Autodesk Inventor part; units mm, degrees
ref_plane "YZ Plane" through (0, 0, 0) normal (1, 0, 0) x (0, 1, 0)
ref_plane "XZ Plane" through (0, 0, 0) normal (0, 1, 0) x (-1, 0, 0)
ref_plane "XY Plane" through (0, 0, 0) normal (0, 0, 1) x (1, 0, 0)
sketch "草圖1" plane through (0, 0, 0) normal (0, 0, 1) x (1, 0, 0)
  line L0 (0, -16.62) -> (0, 16.62) construction
  line L1 (2, -16.62) -> (2, 16.62)
  line L2 (-2, 16.62) -> (-2, -16.62)
  arc A0 (-2, -16.62) -> (2, -16.62) centre (0, -16.62) ccw
  arc A1 (2, 16.62) -> (-2, 16.62) centre (0, 16.62) ccw
  point P0 (0, 0)
  dimension "d0" = 33.24
  dimension "d1" = 4
extrude "擠出1" add sketch "草圖1" along normal blind 1
sketch "草圖2" plane through (0, 0, 1) normal (0, 0, 1) x (1, 0, 0)
  arc A0 (2, 16.62) -> (-2, 16.62) centre (0, 16.62) ccw
  circle A1 centre (0, 16.62) radius 0.75
  arc A2 (-2, -16.62) -> (2, -16.62) centre (0, -16.62) ccw
  circle A3 centre (0, -16.62) radius 0.75
  point P0 (0, 0)
  dimension "d4" = 1.5
  dimension "d5" = 1.5
extrude "擠出2" add sketch "草圖2" along normal blind 1
hole "孔1" at (0, -16.62, 1) at (0, 16.62, 1) direction (0, 0, -1) diameter 2 end through all
hole "孔2" at (0, -16.62, 1) at (0, 16.62, 1) direction (0, 0, 1) diameter 2 end through all
properties part number "連桿4"
Design review of the part built by this model. Coordinates are the model's own, in mm. Round coordinates to 2 decimals unless told otherwise and drop trailing zeros. Order: outer loops, then holes, each group sorted by start corner. A loop starts at its lowest first (then second) coordinate and runs counter-clockwise, first axis right, second up. Notation, with made-up numbers: (52.25, 69.5) - (80.25, 69.5) arc R17 ccw to (80.25, 94.5) - close; hole circle Ø9 at (61.25, -22.5). An arc over 180 degrees is marked (long way). Return JSON: item names as keys, results as strings.
Q1. Wall thickness on L1, parallel to Y at x = 0, z = 0.2; L2, parallel to Y at x = 0.25, z = 0.4; L3, parallel to X at y = 16.62, z = 0.5: over which ranges is each line inside the solid? List them lowest first. Write a range as [from, to].
Computed values:
{"L1": "y = [-18.62, -17.62], [-15.62, 15.62], [17.62, 18.62]", "L2": "y = [-18.6, -17.59], [-15.65, 15.65], [17.59, 18.6]", "L3": "x = [-2, -1], [1, 2]"}
Q2. Consider section A-A on x = 0. Write out the cut boundary in (y, z).
Computed values:
{"outline": "(-18.62, 0) - (-17.62, 0) - (-17.62, 1) - (-18.62, 1) - close; (-15.62, 0) - (15.62, 0) - (15.62, 1) - (-15.62, 1) - close; (17.62, 0) - (18.62, 0) - (18.62, 1) - (17.62, 1) - close"}
Q3. Consider section B-B on z = 0.2. Write out the cut boundary in (x, y), plus the area to 3 significant figures.
Computed values:
{"outline": "(-2, -16.62) arc R2 ccw to (2, -16.62) - (2, 16.62) arc R2 ccw to (-2, 16.62) - close; hole circle Ø2 at (0, -16.62); hole circle Ø2 at (0, 16.62)", "area": "139 mm2"}
Q4. The part is to be moulded in two halves that separate along Y. For faces 1 (the flat face through (-2, 0.2, 0.5)), 2 (the cylindrical face through (0.383, -17.544, 0.493)), 3 (the cylindrical face through (0.04, -18.62, 0.49)), 4 (the cylindrical face through (-0.04, 18.62, 0.49)), say which applies: pulls with the +Y half, pulls with the -Y half, needs draft (parallel to the pull), parting line crosses it, or undercut.
Computed values:
{"face 1": "needs draft", "face 2": "undercut", "face 3": "pulls with the -Y half", "face 4": "pulls with the +Y half"}
